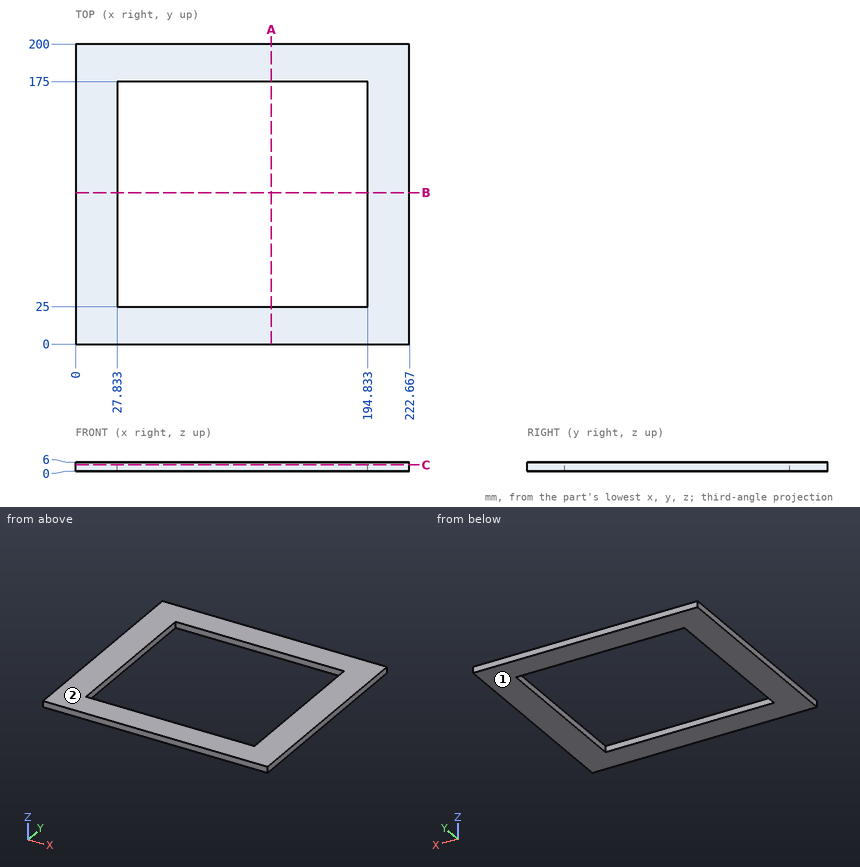
For this review, use the dimensioned drawing (mm, ordinates from the lowest corner) and the shaded views. Round coordinates to 2 decimals unless told otherwise and drop trailing zeros. Write each loop counter-clockwise with the first axis right and the second up, starting at its lowest first coordinate (ties: lowest second). Pieces come first, ordered by that corner, then holes. Notation, with made-up numbers: (41, -30.5) - (92, -30.5) arc R21 cw to (92, -24.5) - close; hole circle Ø1 at (-33, 23.25). An arc over 180 degrees is marked (long way). One line per item, written item: value. Start each with the question number.
1. Consider section B-B on y = 101. Write out the cut boundary in (x, z), and give its area (3 significant figures).
2. Consider section A-A on x = 130.5. Write out the cut boundary in (y, z).
3. The part is to be moulded in two halves that separate along Z. For the marked faces 1 and 2, say which applies: released by +Z, released by -Z, zero draft, split by the parting line, or undercut.
4. To check wall thickness, follow L1, parallel to Y at x = 65.5, z = 3.25; L2, parallel to X at y = 172, z = 0.95. State the ranges of each line that lie inside material, in increasing order. Write a range as from..to.
5. Consider section C-C on z = 4.05. Write out the cut boundary in (x, y), and give its area (3 significant figures).
Checks:
1. outline: (0, 0) - (27.83, 0) - (27.83, 6) - (0, 6) - close; (194.83, 0) - (222.67, 0) - (222.67, 6) - (194.83, 6) - close
1. area: 334 mm^2
2. outline: (0, 0) - (25, 0) - (25, 6) - (0, 6) - close; (175, 0) - (200, 0) - (200, 6) - (175, 6) - close
3. face 1: released by -Z
3. face 2: released by +Z
4. L1: y = 0..25, 175..200
4. L2: x = 0..27.83, 194.83..222.67
5. outline: (0, 0) - (222.67, 0) - (222.67, 200) - (0, 200) - close; hole (27.83, 25) - (194.83, 25) - (194.83, 175) - (27.83, 175) - close
5. area: 19,500 mm^2
